Geometry check sheet. Reference: the model listing, model coordinates, mm. A direction names the side the tool comes from. Give positions to 0.01 mm unless a question says otherwise; leave off trailing zeros. Loops run counter-clockwise (first coordinate to the right, second up) from the corner with the lowest first, then second, coordinate; pieces in that order, holes last. Notation, with made-up numbers: (73.5, -15) - (119.5, -15) arc R27 cw to (119.5, 17) - close; hole circle Ø6 at (-36, -23.75). An arc over 180 degrees is marked (long way). Use a Markdown table: item, result. Add a question column.
1. Set-up check for faces 1 (the cylindrical face through (8.2, 16, -0.5)), 2 (the flat face through (2, 18.5, 3)), 3 (the cylindrical face through (-5.323, 3.944, 2.769)): record each of +Z, -Z, +X, -X, +Y, -Y from which the full face is reachable in a straight line by a thin tool's end or side.
2. Draft check along Y on faces 4 (the cylindrical face through (4.041, 2.633, 0.303)), 5 (the cylindrical face through (1.802, 13.246, 5.723)), 6 (the flat face through (0, 0, 3)), 7 (the cylindrical face through (-4.55, 10.46, -7.13)). Enter one of: pulls with the +Y half, pulls with the -Y half, needs draft (parallel to the pull), parting line crosses it, or undercut.
3. Material ranges on L1, parallel to Y at x = -3.75, z = 0; L2, parallel to X at y = 12, z = 1.5; L3, parallel to Z at x = -5, y = 4, recorded low to high.
4. Cross-section at B-B on z = 0. Enter the section's corners in (x, y), and give its area (3 significant figures).
5. Cross-section at A-A on y = 3.25. Enter the section's corners in (x, z), and give its area (3 significant figures).
6. Cross-section at D-D on x = 4.25. Enter the section's corners in (y, z), and give its area (3 significant figures).
7. Depth check by flat-ended pin: P1, Ø1, axis at y = 11.5, z = 0, coming from the +X side; P2, Ø2.5, axis at y = 4, z = 0, coming from the -X side; P3, Ø1.5, axis at y = 9.5, z = -6, coming from the +X side; P4, Ø6, axis at y = 2.5, z = 2.5, coming from the +X side. Enter the tip coordinate at first touch or a pass-through.
8. Cross-section at C-C on x = -1. Enter the section's corners in (y, z).
from build123d import *

# Parameters (mm, degrees)
SKETCH2_R              = 6
BASE_DEPTH             = 8
SKETCH3_R              = 7.475
CAM_A_DEPTH            = 5
SKETCH4_R              = 6
SPACER_DEPTH           = 0.5
SKETCH5_R              = 7.475
CAM_B_DEPTH            = 5
SKETCH6_R              = 2.55
SHAFT_HOLE_DEPTH       = 23.0907904
SCREW_HOLES_DEPTH      = 23.0907904
SCREW_HOLES_DEPTH_BACK = 23.0907904
SKETCH7_R              = 1.4


with BuildPart() as part:
    # Sketch2 → Base (new body)
    with BuildSketch(Plane(origin=(0, 0, 0), x_dir=(1, 0, 0), z_dir=(0, 1, 0))):
        with Locations(Location((0, 0, 0), (0, 0, 270))):
            Circle(SKETCH2_R)
    extrude(amount=BASE_DEPTH)

    # Sketch3 → Cam A (add)
    with BuildSketch(Plane(origin=(0, 8, 0), x_dir=(1, 0, 0), z_dir=(0, 1, 0))):
        with Locations(Location((0, 1.2, 0), (0, 0, 270))):
            Circle(SKETCH3_R)
    extrude(amount=CAM_A_DEPTH)

    # Sketch4 → Spacer (add)
    with BuildSketch(Plane(origin=(0, 13, 0), x_dir=(1, 0, 0), z_dir=(0, 1, 0))):
        with Locations(Location((0, 0, 0), (0, 0, 270))):
            Circle(SKETCH4_R)
    extrude(amount=SPACER_DEPTH)

    # Sketch5 → Cam B (add)
    with BuildSketch(Plane(origin=(0, 13.5, 0), x_dir=(1, 0, 0), z_dir=(0, 1, 0))):
        with Locations(Location((0.921272716, -1.2, 0), (0, 0, 116.029296009))):
            Circle(SKETCH5_R)
    extrude(amount=CAM_B_DEPTH)

    # Sketch6 → Shaft Hole (cut, through all)
    with BuildSketch(Plane(origin=(0, 18.5, 0), x_dir=(1, 0, 0), z_dir=(0, 1, 0))):
        with Locations(Location((0, 0, 0), (0, 0, 270))):
            Circle(SKETCH6_R)
    extrude(amount=-SHAFT_HOLE_DEPTH, mode=Mode.SUBTRACT)

    # Sketch7 → Screw Holes (cut, two sides: drawn at the far end of the back side and taken through both)
    with BuildSketch(Plane(origin=(0, 0, 0), x_dir=(0, 0, -1), z_dir=(1, 0, 0)).offset(-SCREW_HOLES_DEPTH_BACK)):
        with Locations((0, 4)):
            Circle(SKETCH7_R)
    extrude(amount=SCREW_HOLES_DEPTH + SCREW_HOLES_DEPTH_BACK, mode=Mode.SUBTRACT)


solid = part.part
Values found:
| question | item | result |
|---|---|---|
| 1 | face 1 | +Y |
| 1 | face 2 | +Z, -Z, +X, -X, +Y |
| 1 | face 3 | -Y |
| 2 | face 4 | undercut |
| 2 | face 5 | undercut |
| 2 | face 6 | pulls with the -Y half |
| 2 | face 7 | needs draft |
| 3 | L1 | y = 0 to 2.6, 5.4 to 18.5 |
| 3 | L2 | x = -6.97 to -2.06, 2.06 to 6.97 |
| 3 | L3 | z = -3.32 to -1.4, 1.4 to 3.32 |
| 4 | outline | (-7.38, 8) - (-6, 8) - (-6, 5.4) - (-2.55, 5.4) - (-2.55, 18.5) - (-6.46, 18.5) - (-6.46, 13.5) - (-6, 13.5) - (-6, 13) - (-7.38, 13) - close; (-6, 0) - (-2.55, 0) - (-2.55, 2.6) - (-6, 2.6) - close; (2.55, 0) - (6, 0) - (6, 2.6) - (2.55, 2.6) - close; (2.55, 5.4) - (6, 5.4) - (6, 8) - (7.38, 8) - (7.38, 13) - (6, 13) - (6, 13.5) - (8.3, 13.5) - (8.3, 18.5) - (2.55, 18.5) - close |
| 4 | area | 136 mm2 |
| 5 | outline | (-5.88, -1.18) arc R6 ccw to (5.88, -1.18) - (2.26, -1.18) arc R2.55 cw to (-2.26, -1.18) - close; (-5.88, 1.18) - (-2.26, 1.18) arc R2.55 cw to (2.26, 1.18) - (5.88, 1.18) arc R6 ccw to start |
| 5 | area | 76.1 mm2 |
| 6 | outline | (0, -4.24) - (8, -4.24) - (8, -7.35) - (13, -7.35) - (13, -4.24) - (13.5, -4.24) - (13.5, -5.49) - (18.5, -5.49) - (18.5, 7.89) - (13.5, 7.89) - (13.5, 4.24) - (13, 4.24) - (13, 4.95) - (8, 4.95) - (8, 4.24) - (0, 4.24) - close; hole circle Ø2.8 at (4, 0) |
| 6 | area | 194 mm2 |
| 7 | P1 | stops at x = 7.44 |
| 7 | P2 | passes through |
| 7 | P3 | stops at x = 6.28 |
| 7 | P4 | stops at x = 6 |
| 8 | outline | (0, -5.92) - (8, -5.92) - (8, -8.61) - (13, -8.61) - (13, -5.92) - (13.5, -5.92) - (13.5, -6.02) - (18.5, -6.02) - (18.5, -2.35) - (0, -2.35) - close; (0, 2.35) - (18.5, 2.35) - (18.5, 8.42) - (13.5, 8.42) - (13.5, 5.92) - (13, 5.92) - (13, 6.21) - (8, 6.21) - (8, 5.92) - (0, 5.92) - close |
